Source: CAD feature listing. Evaluate the final solid. Frame: model axes, mm. A direction names the side the tool comes from. Round coordinates to 2 decimals unless told otherwise and drop trailing zeros. Write each loop counter-clockwise with the first axis right and the second up, starting at its lowest first coordinate (ties: lowest second). Pieces come first, ordered by that corner, then holes. Notation, with made-up numbers: M 20.25,53 L 48.25,53 A14 ccw 48.25,79 Z; hole C 83.5,56 d11. An arc over 180 degrees is marked long. Answer in a Markdown table with one row per item.
from build123d import *

# Parameters (mm, degrees)
SKETCH_1_W          = 14
SKETCH_1_H          = 14
SKETCH_1_W_2        = 12
SKETCH_1_H_2        = 12
EXTRUDE_1_DEPTH     = 14
EXTRUDE_3_DEPTH     = 14
SKETCH_3_W          = 10
SKETCH_3_H          = 10
CUT_EXTRUDE_1_DEPTH = 10


with BuildPart() as part:
    # 草图1 → 凸台-拉伸1 (new body)
    with BuildSketch(Plane.XY):
        with Locations((7, 7)):
            Rectangle(SKETCH_1_W, SKETCH_1_H)
        with Locations((7, 7)):
            Rectangle(SKETCH_1_W_2, SKETCH_1_H_2, mode=Mode.SUBTRACT)
    extrude(amount=EXTRUDE_1_DEPTH)

    # 草图2 → 凸台-拉伸3 (add)
    with BuildSketch(Plane(origin=(0, 0, 0), x_dir=(-1, 0, 0), z_dir=(0, 0, -1))):
        Polygon((-0.869466018, 29.259809863), (-8.044126787, 20.92169), (0, 14), (2.568025419, 11.790303866), (9.742686188, 20.128423729), align=None)
        Polygon((-13.999999155, 14), (-8.044126787, 20.92169), (0, 14), align=None)
        Polygon((2.568025419, 11.790303866), (0, 14), (0, 8.805841681), align=None)
    extrude(amount=-EXTRUDE_3_DEPTH)

    # 草图3 → 切除-拉伸1 (cut)
    with BuildSketch(Plane(origin=(-14.096351186, 16.382247136, 0), x_dir=(0.75801089666448, 0.6522418880583423, 0), z_dir=(-0.6522418880583423, 0.75801089666448, 0))):
        with Locations((12.743538804, -7)):
            Rectangle(SKETCH_3_W, SKETCH_3_H)
    extrude(amount=-CUT_EXTRUDE_1_DEPTH, mode=Mode.SUBTRACT)


solid = part.part
Q1. Section A-A (y = 8). Return loops of the section in (x, z).
Solutions:
| item | result |
|---|---|
| outline | M 0,0 L 1,0 L 1,14 L 0,14 Z; M 13,0 L 14,0 L 14,14 L 13,14 Z |
Q2. Pull-direction query (Z, two-part tool) for faces 1 (the flat face through (2, 17, 14)), 2 (the flat face through (-1, 21, 2)), 3 (the flat face through (13, 7, 7)); classes: pulls with the +Z half, pulls with the -Z half, needs draft (parallel to the pull), parting line crosses it, or undercut.
Solutions:
| item | result |
|---|---|
| face 1 | pulls with the +Z half |
| face 2 | undercut |
| face 3 | needs draft |
Q3. Section C-C (x = 1.5). Return loops of the section in (y, z).
Solutions:
| item | result |
|---|---|
| outline | M 0,0 L 1,0 L 1,14 L 0,14 Z; M 13,0 L 28.53,0 L 28.53,14 L 13,14 Z; hole M 16.61,2 L 25.46,2 L 25.46,12 L 16.61,12 Z |
Q4. Material intervals for probe 1 along X at (y, z) = (8, 12); probe 2 along Z at (x, y) = (1.5, 19); probe 3 along Y at (x, z) = (2.75, 9.5), sorted ascending.
Solutions:
| item | result |
|---|---|
| probe 1 | x = 0 to 1, 13 to 14 |
| probe 2 | z = 0 to 2, 12 to 14 |
| probe 3 | y = 0 to 1, 13 to 17.69, 24.01 to 27.07 |
Q5. Contact query for flat-ended pins moving along their axis: pin 1 Ø6 at (x, y) = (-5.5, 4.5) entering from -Z; pin 2 Ø7 at (x, y) = (-2.5, 22) entering from -Z; pin 3 Ø3.5 at (y, z) = (5, 5) entering from -X; pin 4 Ø1.5 at (y, z) = (21.5, 6.5) entering from +X. Output: stop coordinate, or through.
Solutions:
| item | result |
|---|---|
| pin 1 | passes through |
| pin 2 | stops at z = 0 |
| pin 3 | stops at x = 0 |
| pin 4 | stops at x = 8.19 |
Q6. Access query for faces 4 (the flat face through (0, 4, 7)), 5 (the flat face through (2.033, 17.068, 6.93)), 6 (the flat face through (7, 13, 7)). Directions: +Z, -Z, +X, -X, +Y, -Y. A direction counts if a zero-diameter tool reaches every point of the face in a straight line with its end or side. Return the directions, or none.
Solutions:
| item | result |
|---|---|
| face 4 | +Z, -Z, -X, -Y |
| face 5 | none |
| face 6 | +Z, -Z |
Q7. Section D-D (x = 11.75). Return loops of the section in (y, z).
Solutions:
| item | result |
|---|---|
| outline | M 0,0 L 1,0 L 1,14 L 0,14 Z; M 13,0 L 16.61,0 L 16.61,14 L 13,14 Z |
